from build123d import *

# Parameters (mm, degrees)
F0_W     = 1930.4
F0_H     = 254
F1_DEPTH = 12.7
F3_DEPTH = 12.7


# Not quite as in the source:
# - ends of sketch curves that miss each other by under 0.0002 mm in the source are joined
# - a feature names something its author has since deleted; it is built from what else it names


with BuildPart() as f1:
    # F0 (on Top) → F1 (new body)
    with BuildSketch(Plane.XY):
        with Locations((-75.096349721, -133.9091630952)):
            Rectangle(F0_W, F0_H)
        with BuildLine():
            ThreePointArc((-862.496349721, -159.3091630952), (-887.896349721, -133.9091630952), (-862.496349721, -108.5091630952))
            Line((-862.496349721, -108.5091630952), (712.303650279, -108.5091630952))
            ThreePointArc((712.303650279, -108.5091630952), (737.703650279, -133.9091630952), (712.303650279, -159.3091630952))
            Line((712.303650279, -159.3091630952), (-862.496349721, -159.3091630952))
        make_face(mode=Mode.SUBTRACT)
    extrude(amount=F1_DEPTH)

    # F2 (on face) + F0 (on Top) → F3 (join)
    with BuildSketch(Plane(origin=(0, 0, 0), x_dir=(1, 0, 0), z_dir=(0, 0, -1))):
        with BuildLine():
            ThreePointArc((-506.896349721, 159.3091630952), (-481.496349721, 133.9091630952), (-506.896349721, 108.5091630952))
            Line((-506.896349721, 108.5091630952), (-411.646349721, 108.5091630952))
            ThreePointArc((-411.646349721, 108.5091630952), (-437.046349721, 133.9091630952), (-411.646349721, 159.3091630952))
            Line((-411.646349721, 159.3091630952), (-506.896349721, 159.3091630952))
        make_face()
        with BuildLine():
            ThreePointArc((261.453650279, 159.3091630952), (286.853650279, 133.9091630952), (261.453650279, 108.5091630952))
            Line((261.453650279, 108.5091630952), (356.703650279, 108.5091630952))
            ThreePointArc((356.703650279, 108.5091630952), (331.303650279, 133.9091630952), (356.703650279, 159.3091630952))
            Line((356.703650279, 159.3091630952), (261.453650279, 159.3091630952))
        make_face()
    with BuildSketch(Plane.XY):
        with Locations((-75.096349721, -133.9091630952)):
            Rectangle(F0_W, F0_H)
        with BuildLine():
            ThreePointArc((-862.496349721, -159.3091630952), (-887.896349721, -133.9091630952), (-862.496349721, -108.5091630952))
            Line((-862.496349721, -108.5091630952), (712.303650279, -108.5091630952))
            ThreePointArc((712.303650279, -108.5091630952), (737.703650279, -133.9091630952), (712.303650279, -159.3091630952))
            Line((712.303650279, -159.3091630952), (-862.496349721, -159.3091630952))
        make_face(mode=Mode.SUBTRACT)
    extrude(amount=F3_DEPTH, dir=(0, 0, -1))


solid = f1.part
For this review, take the finished solid that the model builds, in its own axes (mm). A direction names the side the tool comes from. Round coordinates to 2 decimals unless told otherwise and drop trailing zeros. Order: outer loops, then holes, each group sorted by start corner. A loop starts at its lowest first (then second) coordinate and runs counter-clockwise, first axis right, second up. Notation, with made-up numbers: M 52,-16 L 67,-16 A30 ccw 67,23 Z; hole C -34,83.25 d11. An arc over 180 degrees is marked long. Write each question's results on one line, items separated by ' | '. Start each with the question number.
1. Add section A-A (x = 220). State the section outline as (y, z) points, then the cut area to 3 significant figures.
2. Draft analysis for pull direction X (two halves, no side actions). For faces 3 (the face through (-89, -104, -12.7)), 4 (the face through (-460, -134, 0)), state which applies: pulls with the +X half, pulls with the -X half, needs draft (parallel to the pull), parting line crosses it, or undercut.
3. Add section B-B (z = 5.25). State the section outline as (x, y) points, then the cut area to 3 significant figures.
4. Tool access review of faces 1 (the face through (-89, -160, 12.7)), 2 (the face through (308, -134, 0)): name each direction out of +Z, -Z, +X, -X, +Y, -Y from which nothing blocks a thin tool from reaching the whole face with its end or side.
5. To check wall thickness, follow L1, parallel to Y at x = -603.5, z = -10; L2, parallel to X at y = -140, z = 9.25; L3, parallel to X at y = -115.5, z = 10.5. State the ranges of each line that lie inside material, in increasing order. Write a range as [from, to].
Output values:
1) outline: M -260.91,-12.7 L -159.31,-12.7 L -159.31,12.7 L -260.91,12.7 Z; M -108.51,-12.7 L -6.91,-12.7 L -6.91,12.7 L -108.51,12.7 Z | area: 5,160 mm^2
2) face 3: needs draft | face 4: undercut
3) outline: M -1040.3,-260.91 L 890.1,-260.91 L 890.1,-6.91 L -1040.3,-6.91 Z; hole M -862.5,-159.31 L 712.3,-159.31 A25.4 ccw 712.3,-108.51 L -862.5,-108.51 A25.4 ccw Z | area: 408,000 mm^2
4) face 1: +Z, +X, -X, +Y, -Y | face 2: +Z
5) L1: [-260.91, -159.31], [-108.51, -6.91] | L2: [-1040.3, -887.16], [736.96, 890.1] | L3: [-1040.3, -880], [729.8, 890.1]
